For this review, take the finished solid that the model builds, in its own axes (mm). A direction names the side the tool comes from. Give positions to 0.01 mm unless a question says otherwise; leave off trailing zeros. Loops run counter-clockwise (first coordinate to the right, second up) from the corner with the lowest first, then second, coordinate; pieces in that order, holes last.
```python
from build123d import *

# Parameters (mm, degrees)
BOSS_EXTRUDE1_DEPTH = 6
BOSS_EXTRUDE2_DEPTH = 3
SKETCH3_R           = 1.6
CUT_EXTRUDE1_DEPTH  = 67.155290794
CHAMFER1_SIZE       = 1.3
FILLET1_R           = 1.5


with BuildPart() as part:
    # Sketch1 → Boss-Extrude1 (new body)
    with BuildSketch(Plane.XY):
        with BuildLine():
            Line((-23.3, 50.5), (-23.3, 2.2))
            Line((-23.3, 2.2), (23.3, 2.2))
            Line((23.3, 2.2), (23.3, 50.5))
            ThreePointArc((23.3, 50.5), (21.89411255, 53.89411255), (18.5, 55.3))
            Line((18.5, 55.3), (-18.5, 55.3))
            ThreePointArc((-18.5, 55.3), (-21.89411255, 53.89411255), (-23.3, 50.5))
        make_face()
    extrude(amount=-BOSS_EXTRUDE1_DEPTH)

    # Sketch2 → Boss-Extrude2 (add)
    with BuildSketch(Plane.XY):
        with BuildLine():
            Line((-25.6, 11.2), (-32.35, 2.2))
            Line((-32.35, 2.2), (-23.3, 2.2))
            Line((-23.3, 2.2), (23.3, 2.2))
            Line((23.3, 2.2), (32.35, 2.2))
            Line((32.35, 2.2), (25.6, 11.2))
            ThreePointArc((25.6, 11.2), (25.153950106, 12.051316702), (25, 13))
            Line((25, 13), (25, 52))
            ThreePointArc((25, 52), (23.535533906, 55.535533906), (20, 57))
            Line((20, 57), (-20, 57))
            ThreePointArc((-20, 57), (-23.535533906, 55.535533906), (-25, 52))
            Line((-25, 52), (-25, 13))
            ThreePointArc((-25, 13), (-25.153950106, 12.051316702), (-25.6, 11.2))
        make_face()
    extrude(amount=BOSS_EXTRUDE2_DEPTH)

    # Sketch3 → Cut-Extrude1 (cut, through all)
    with BuildSketch(Plane.XY.offset(3)):
        with Locations((-26.5, 5)):
            Circle(SKETCH3_R)
        with Locations((26.5, 5)):
            Circle(SKETCH3_R)
    extrude(amount=-CUT_EXTRUDE1_DEPTH, mode=Mode.SUBTRACT)

    # Chamfer1
    # the kernel refuses this chamfer: 1.3 mm, written as the material it takes off along each edge
    with BuildSketch(Plane(origin=(-26.5, 5, 3), x_dir=(1, 0, 0), z_dir=(0, -1, 0))) as chamfer1_piece_1:
        Polygon((1.6 + CHAMFER1_SIZE, 0), (1.6, -CHAMFER1_SIZE), (1.6, 0), align=None)
    revolve(axis=Axis((-26.5, 5, 3), (0, 0, 1)), mode=Mode.SUBTRACT)
    with BuildSketch(Plane(origin=(26.5, 5, 3), x_dir=(1, 0, 0), z_dir=(0, -1, 0))) as chamfer1_piece_2:
        Polygon((1.6 + CHAMFER1_SIZE, 0), (1.6, -CHAMFER1_SIZE), (1.6, 0), align=None)
    revolve(axis=Axis((26.5, 5, 3), (0, 0, 1)), mode=Mode.SUBTRACT)

    # Fillet1
    # the kernel refuses this fillet: 1.5 mm, written as the material it takes off along each edge
    with BuildSketch(Plane(origin=(-28, 13, 3), x_dir=(1, 0, 0), z_dir=(0, 1, 0))) as fillet1_piece_1:
        with BuildLine():
            CenterArc((3 + FILLET1_R, FILLET1_R), FILLET1_R, 180, 90)
            Line((3 + FILLET1_R, 0), (3, 0))
            Line((3, 0), (3, FILLET1_R))
        make_face()
    revolve(axis=Axis((-28, 13, 3), (0, 0, -1)), revolution_arc=36.869897646, mode=Mode.SUBTRACT)
    with BuildSketch(Plane(origin=(-25.6, 11.2, 3), x_dir=(0, 0, -1), z_dir=(-0.6000000000000002, -0.7999999999999998, 0))) as fillet1_piece_2:
        with BuildLine():
            CenterArc((FILLET1_R, FILLET1_R), FILLET1_R, 180, 90)
            Line((0, FILLET1_R), (0, 0))
            Line((0, 0), (FILLET1_R, 0))
        make_face()
    extrude(amount=15, mode=Mode.SUBTRACT)
    with BuildSketch(Plane(origin=(34.6, -0.8, 3), x_dir=(-0.800000000000001, -0.5999999999999985, 0), z_dir=(-0.5999999999999985, 0.8000000000000012, 0))) as fillet1_piece_3:
        with BuildLine():
            CenterArc((FILLET1_R, -FILLET1_R), FILLET1_R, 90, 90)
            Line((0, -FILLET1_R), (0, 0))
            Line((0, 0), (FILLET1_R, 0))
        make_face()
    extrude(amount=15, mode=Mode.SUBTRACT)
    with BuildSketch(Plane(origin=(28, 13, 3), x_dir=(-0.8000000000000014, -0.5999999999999981, 0), z_dir=(0.5999999999999981, -0.8000000000000014, 0))) as fillet1_piece_4:
        with BuildLine():
            CenterArc((3 + FILLET1_R, FILLET1_R), FILLET1_R, 180, 90)
            Line((3, FILLET1_R), (3, 0))
            Line((3, 0), (3 + FILLET1_R, 0))
        make_face()
    revolve(axis=Axis((28, 13, 3), (0, 0, -1)), revolution_arc=36.869897646, mode=Mode.SUBTRACT)
    with BuildSketch(Plane(origin=(25, 13, 3), x_dir=(-1, 0, 0), z_dir=(0, 1, 0)), Plane(origin=(-25, 52, 3), x_dir=(1, 0, 0), z_dir=(0, -1, 0))) as fillet1_piece_5:
        with BuildLine():
            CenterArc((FILLET1_R, -FILLET1_R), FILLET1_R, 90, 90)
            Line((0, -FILLET1_R), (0, 0))
            Line((0, 0), (FILLET1_R, 0))
        make_face()
    extrude(amount=39, mode=Mode.SUBTRACT)
    with BuildSketch(Plane(origin=(20, 52, 3), x_dir=(1, 0, 0), z_dir=(0, -1, 0))) as fillet1_piece_6:
        with BuildLine():
            CenterArc((5 - FILLET1_R, -FILLET1_R), FILLET1_R, 0, 90)
            Line((5, -FILLET1_R), (5, 0))
            Line((5, 0), (5 - FILLET1_R, 0))
        make_face()
    revolve(axis=Axis((20, 52, 3), (0, 0, 1)), revolution_arc=90, mode=Mode.SUBTRACT)
    with BuildSketch(Plane(origin=(20, 57, 3), x_dir=(0, -1, 0), z_dir=(-1, 0, 0))) as fillet1_piece_7:
        with BuildLine():
            CenterArc((FILLET1_R, -FILLET1_R), FILLET1_R, 90, 90)
            Line((0, -FILLET1_R), (0, 0))
            Line((0, 0), (FILLET1_R, 0))
        make_face()
    extrude(amount=40, mode=Mode.SUBTRACT)
    with BuildSketch(Plane(origin=(-20, 52, 3), x_dir=(0, 1, 0), z_dir=(1, 0, 0))) as fillet1_piece_8:
        with BuildLine():
            CenterArc((5 - FILLET1_R, -FILLET1_R), FILLET1_R, 0, 90)
            Line((5, -FILLET1_R), (5, 0))
            Line((5, 0), (5 - FILLET1_R, 0))
        make_face()
    revolve(axis=Axis((-20, 52, 3), (0, 0, 1)), revolution_arc=90, mode=Mode.SUBTRACT)


solid = part.part
```
Item 1: Take a section at B-B on z = -2.75. Give the boundary of the cut face in (x, y).
Answer:
outline: (-23.3, 2.2) - (23.3, 2.2) - (23.3, 50.5) arc R4.8 ccw to (18.5, 55.3) - (-18.5, 55.3) arc R4.8 ccw to (-23.3, 50.5) - close
Item 2: Clearance check with flat-ended pins moving along their axes: pin 1 Ø2 at (y, z) = (45, -1.5) entering from -X; pin 2 Ø2.5 at (x, y) = (26.5, 5) entering from -Z; pin 3 Ø3 at (y, z) = (23.5, -2.5) entering from +X; pin 4 Ø0.8 at (y, z) = (27, 0.5) entering from -X. State where each tip first meets the part, or that it passes through.
Answer:
pin 1: stops at x = -23.3
pin 2: passes through
pin 3: stops at x = 23.3
pin 4: stops at x = -25
Item 3: Take a section at C-C on y = 17. Give the boundary of the cut face in (x, z).
Answer:
outline: (-25, 0) - (-23.3, 0) - (-23.3, -6) - (23.3, -6) - (23.3, 0) - (25, 0) - (25, 1.5) arc R1.5 ccw to (23.5, 3) - (-23.5, 3) arc R1.5 ccw to (-25, 1.5) - close
Item 4: Take a section at A-A on x = -14. Give the boundary of the cut face in (y, z), and give its area (3 significant figures).
Answer:
outline: (2.2, -6) - (55.3, -6) - (55.3, 0) - (57, 0) - (57, 1.5) arc R1.5 ccw to (55.5, 3) - (2.2, 3) - close
area: 483 mm2
Item 5: Take a section at D-D on y = 5. State how many separate pieces and enclosed holes the cut face has, and give its area (3 significant figures).
Answer:
separate pieces: 3
enclosed holes: 0
area: 437 mm2
Item 6: The part is to be moulded in two halves that separate along Y. For faces 1 (the cylindrical face through (25.23, 4.03, 0.86)), 2 (the cylindrical face through (25.158, 12.039, 0.74)), 3 (the flat face through (0, 29, -6)), say which applies: released by +Y, released by -Y, zero draft, split by the parting line, or undercut.
Answer:
face 1: undercut
face 2: released by +Y
face 3: zero draft
Item 7: Tool access review of faces 4 (the cylindrical face through (21.93, 53.86, -2.96)), 5 (the cylindrical face through (-24.55, 32.77, 2.57)), 6 (the flat face through (-25, 33, 1)), 7 (the flat face through (23.3, 26, -3)), 8 (the cylindrical face through (-21.86, 53.93, -2.96)): name each direction out of +Z, -Z, +X, -X, +Y, -Y from which nothing blocks a thin tool from reaching the whole face with its end or side.
Answer:
face 4: -Z, +X, +Y
face 5: +Z, -X, +Y
face 6: +Z, -Z, -X, +Y
face 7: -Z, +X, +Y, -Y
face 8: -Z, -X, +Y
Item 8: For L1, parallel to Y at x = -4, z = -1.5; L2, parallel to X at y = 20, z = -4.25; L3, parallel to X at y = 19.5, z = 1, list the stretches that pass through material, from the lowest coordinate up.
Answer:
L1: y = 2.2 to 55.3
L2: x = -23.3 to 23.3
L3: x = -25 to 25
